Read the model definition and answer for the solid it produces. Units are mm, in the model's axes. Face numbers are marked on the shaded views. A direction names the side the tool comes from. Round coordinates to 2 decimals unless told otherwise and drop trailing zeros. Write each loop counter-clockwise with the first axis right and the second up, starting at its lowest first coordinate (ties: lowest second). Pieces come first, ordered by that corner, then holes. Notation, with made-up numbers: (34.5, 36) - (74.5, 36) arc R8 cw to (74.5, 46) - close; hole circle Ø9 at (-13.5, 32). An arc over 180 degrees is marked (long way). One line per item, written item: value. Start each with the question number.
(1) Flat-ended cylindrical pins translate along their axes: pin 1 Ø4 at (x, z) = (-257.5, 42) entering from -Y; pin 2 Ø6 at (x, y) = (-27.5, 63) entering from +Z; pin 3 Ø4.5 at (y, z) = (-60, 24.5) entering from -X. Find the tip coordinate at first contact, or state that the pin passes through.
(2) For the marked faces 1 and 2, determine the directions among +Z, -Z, +X, -X, +Y, -Y from which every point of the face is accessible in a straight line to the end or side of a thin tool.
(3) Find the intervals of material crossed by L1, parallel to Y at x = -325.75, z = 24.5; L2, parallel to Y at x = 267, z = 40.5 (3 decimals); L3, parallel to Z at x = 321, y = 60, in increasing order.
(4) A cutting plane is placed at A-A, the plane y = -18.5. Determine the outline of the cut face in (x, z), plus the area to 3 significant figures.
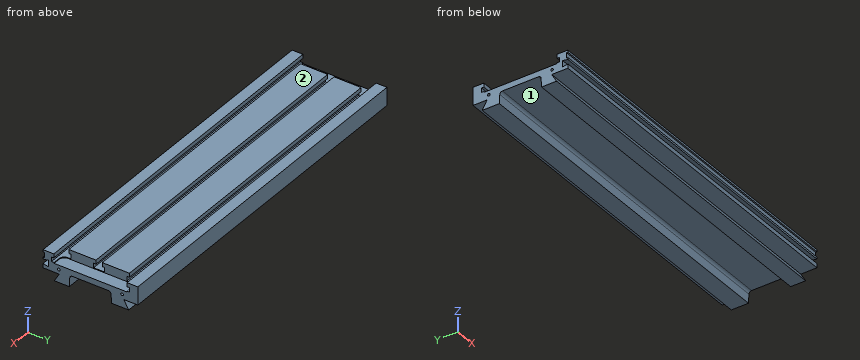
from build123d import *

# Parameters (mm, degrees)
F1_DEPTH      = 337.5
F3_DEPTH      = 1.5
F3_DEPTH_BACK = 16
F5_D          = 5
F5_DEPTH      = 21
F5_TIP        = 1.5021515476
F7_D          = 5
F7_DEPTH      = 21
F7_TIP        = 1.5021515476


with BuildPart() as f1:
    # F0 (on Right) → F1 (new body, symmetric)
    with BuildSketch(Plane.YZ):
        with BuildLine():
            Line((-87.5, 36), (-90, 36))
            Line((-90, 36), (-90, 32.3))
            Line((-90, 32.3), (-80, 34.15))
            Line((-80, 34.15), (-80, 22.15))
            Line((-80, 22.15), (-90, 24))
            Line((-90, 24), (-90, 16))
            Line((-90, 16), (-59.25, 16))
            Line((-59.25, 16), (-68.487604307, 0))
            Line((-68.487604307, 0), (-40, 0))
            Line((-40, 0), (-39.2217531629, 16.7323069968))
            ThreePointArc((-39.2217531629, 16.7323069968), (-37.6795768821, 20.1167343684), (-34.2271527326, 21.5))
            Line((-34.2271527326, 21.5), (34.2271527326, 21.5))
            ThreePointArc((34.2271527326, 21.5), (37.6795768821, 20.1167343684), (39.2217531629, 16.7323069968))
            Line((39.2217531629, 16.7323069968), (40, 0))
            Line((40, 0), (72.487604307, 0))
            Line((72.487604307, 0), (63.25, 16))
            Line((63.25, 16), (90, 16))
            Line((90, 16), (90, 50))
            Line((90, 50), (69.5, 50))
            Line((69.5, 50), (69.5, 42.5))
            Line((69.5, 42.5), (73.875, 42.5))
            Line((73.875, 42.5), (73.875, 34))
            Line((73.875, 34), (53.125, 34))
            Line((53.125, 34), (53.125, 42.5))
            Line((53.125, 42.5), (57.5, 42.5))
            Line((57.5, 42.5), (57.5, 50))
            Line((57.5, 50), (6, 50))
            Line((6, 50), (6, 42.5))
            Line((6, 42.5), (10.375, 42.5))
            Line((10.375, 42.5), (10.375, 34))
            Line((10.375, 34), (-10.375, 34))
            Line((-10.375, 34), (-10.375, 42.5))
            Line((-10.375, 42.5), (-6, 42.5))
            Line((-6, 42.5), (-6, 50))
            Line((-6, 50), (-57.5, 50))
            Line((-57.5, 50), (-57.5, 42.5))
            Line((-57.5, 42.5), (-53.125, 42.5))
            Line((-53.125, 42.5), (-53.125, 34))
            Line((-53.125, 34), (-73.875, 34))
            Line((-73.875, 34), (-73.875, 42.5))
            Line((-73.875, 42.5), (-69.5, 42.5))
            Line((-69.5, 42.5), (-69.5, 50))
            Line((-69.5, 50), (-90, 50))
            Line((-90, 50), (-90, 46))
            Line((-90, 46), (-87.5, 46))
            Line((-87.5, 46), (-87.5, 36))
        make_face()
    extrude(amount=F1_DEPTH, both=True)

    # F2 (on face) → F3 (cut, two sides)
    with BuildSketch(Plane.XY.offset(34)) as f3_sk:
        with BuildLine():
            ThreePointArc((314, -59), (316.9289321881, -66.0710678119), (324, -69))
            Line((324, -69), (337.5, -69))
            Line((337.5, -69), (337.5, 69))
            Line((337.5, 69), (324, 69))
            ThreePointArc((324, 69), (316.9289321881, 66.0710678119), (314, 59))
            Line((314, 59), (314, -59))
        make_face()
        with BuildLine():
            ThreePointArc((-324, -69), (-316.9289321881, -66.0710678119), (-314, -59))
            Line((-314, -59), (-314, 59))
            ThreePointArc((-314, 59), (-316.9289321881, 66.0710678119), (-324, 69))
            Line((-324, 69), (-337.5, 69))
            Line((-337.5, 69), (-337.5, -69))
            Line((-337.5, -69), (-324, -69))
        make_face()
    extrude(amount=-F3_DEPTH, mode=Mode.SUBTRACT)
    extrude(f3_sk.sketch, amount=F3_DEPTH_BACK, mode=Mode.SUBTRACT)

    # F5
    with Locations(Plane.YZ.offset(337.5)):
        with Locations((-60, 24.5), (60, 24.5)):
            Hole(F5_D / 2, depth=F5_DEPTH)
            with Locations((0, 0, -(F5_DEPTH + F5_TIP / 2))):  # 118° drill point
                Cone(0, F5_D / 2, F5_TIP, mode=Mode.SUBTRACT)

    # F7
    with Locations(Plane(origin=(-337.5, 0, 0), x_dir=(0, -1, 0), z_dir=(-1, 0, 0))):
        with Locations((-60, 24.5), (60, 24.5)):
            Hole(F7_D / 2, depth=F7_DEPTH)
            with Locations((0, 0, -(F7_DEPTH + F7_TIP / 2))):  # 118° drill point
                Cone(0, F7_D / 2, F7_TIP, mode=Mode.SUBTRACT)


solid = f1.part
Here are the results:
1. pin 1: y = -87.5
1. pin 2: z = 34
1. pin 3: x = -316.35
2. face 1: -Z, +X, -X
2. face 2: +Z, +X, -X, +Y, -Y
3. L1: -80 to -62.5, -57.5 to 57.5, 62.5 to 90
3. L2: -87.5 to -73.875, -53.125 to -10.375, 10.375 to 53.125, 73.875 to 90
3. L3: 0 to 22, 27 to 32.5
4. outline: (-337.5, 21.5) - (337.5, 21.5) - (337.5, 32.5) - (314, 32.5) - (314, 50) - (-314, 50) - (-314, 32.5) - (-337.5, 32.5) - close
4. area: 18,400 mm²
